Read the model definition and answer for the solid it produces. Units are mm, in the model's axes. A direction names the side the tool comes from. Give positions to 0.01 mm unless a question says otherwise; leave off trailing zeros. Order: outer loops, then holes, each group sorted by start corner. A loop starts at its lowest first (then second) coordinate and runs counter-clockwise, first axis right, second up. Notation, with made-up numbers: (72.5, 51.5) -> (116.5, 51.5) arc R21 cw to (116.5, 71.5) -> close; hole circle Ø10 at (-16, 63). An arc over 180 degrees is marked (long way). Use one line per item in the form item = value.
```python
from build123d import *

# Parameters (mm, degrees)
SKETCH1_W                                        = 183.850004878
SKETCH1_H                                        = 82.78473231
BOSS_EXTRUDE1_DEPTH                              = 30
CSK_FOR_M10_FLAT_HEAD_MACHINE_SCREW2_D           = 11
CSK_FOR_M10_FLAT_HEAD_MACHINE_SCREW2_CSINK_D     = 20
CSK_FOR_M10_FLAT_HEAD_MACHINE_SCREW2_CSINK_ANGLE = 80
CBORE_FOR_M8_HEX_HEAD_BOLT1_D                    = 9
CBORE_FOR_M8_HEX_HEAD_BOLT1_CBORE_D              = 18.01
CBORE_FOR_M8_HEX_HEAD_BOLT1_CBORE_DEPTH          = 5.68
MIRROR2_COPY_1_D                                 = 9
MIRROR2_COPY_1_CBORE_D                           = 18.01
MIRROR2_COPY_1_CBORE_DEPTH                       = 5.68
F_20_0MM_START                                   = 20
F_20_0MM_DOWEL_SLOT1_DEPTH                       = 10


# Read off the part's stored shape, not the designer's step: Ø20.0mm Dowel Slot1
with BuildPart() as part:
    # Sketch1 → Boss-Extrude1 (new body)
    with BuildSketch(Plane(origin=(0, 0, 0), x_dir=(1, 0, 0), z_dir=(0, 1, 0))):
        Rectangle(SKETCH1_W, SKETCH1_H)
    extrude(amount=BOSS_EXTRUDE1_DEPTH)

    # CSK for M10 Flat Head Machine Screw2 (through all)
    with Locations(Plane(origin=(0, 30, 0), x_dir=(1, 0, 0), z_dir=(0, 1, 0))):
        with Locations((0, 0)):
            CounterSinkHole(CSK_FOR_M10_FLAT_HEAD_MACHINE_SCREW2_D / 2, CSK_FOR_M10_FLAT_HEAD_MACHINE_SCREW2_CSINK_D / 2, counter_sink_angle=CSK_FOR_M10_FLAT_HEAD_MACHINE_SCREW2_CSINK_ANGLE)

    # CBORE for M8 Hex Head Bolt1 (through all)
    with Locations(Plane(origin=(-73.52781125, 30, -24.202787729), x_dir=(0, 0, 1), z_dir=(0, 1, 0))):
        with Locations((0, 0)):
            cbore_for_m8_hex_head_bolt1 = CounterBoreHole(CBORE_FOR_M8_HEX_HEAD_BOLT1_D / 2, CBORE_FOR_M8_HEX_HEAD_BOLT1_CBORE_D / 2, CBORE_FOR_M8_HEX_HEAD_BOLT1_CBORE_DEPTH)

    # Mirror1: CBORE for M8 Hex Head Bolt1 across plane
    add(cbore_for_m8_hex_head_bolt1.mirror(Plane.XY), mode=Mode.SUBTRACT)

    # Mirror2: CBORE for M8 Hex Head Bolt1 across plane
    add(cbore_for_m8_hex_head_bolt1.mirror(Plane(origin=(0, 0, 0), x_dir=(0, 0, 1), z_dir=(1, 0, 0))), mode=Mode.SUBTRACT)

    # Mirror2 copy 1 (through all)
    with Locations(Plane(origin=(73.52781125, 30, 24.202787729), x_dir=(0, 0, -1), z_dir=(0, 1, 0))):
        with Locations((0, 0)):
            CounterBoreHole(MIRROR2_COPY_1_D / 2, MIRROR2_COPY_1_CBORE_D / 2, MIRROR2_COPY_1_CBORE_DEPTH)

    # Ø20.0mm Dowel Slot1 outline → Ø20.0mm Dowel Slot1 (cut)
    with BuildSketch(Plane(origin=(0, 0, 0), x_dir=(1, 0, 0), z_dir=(0, 1, 0)).offset(F_20_0MM_START)):
        with BuildLine():
            Line((-50, -41.392366155), (50, -41.392366155))
            ThreePointArc((50, -41.392366155), (47.071067812, -34.321298343), (40, -31.392366155))
            Line((40, -31.392366155), (-40, -31.392366155))
            ThreePointArc((-40, -31.392366155), (-47.071067812, -34.321298343), (-50, -41.392366155))
        make_face()
    f_20_0mm_dowel_slot1 = extrude(amount=F_20_0MM_DOWEL_SLOT1_DEPTH, mode=Mode.SUBTRACT)

    # Mirror3: Ø20.0mm Dowel Slot1 across plane
    add(f_20_0mm_dowel_slot1.mirror(Plane.XY), mode=Mode.SUBTRACT)

    # Sketch20 → M12x1.5 Tapped Hole1 (revolve, cut)
    with BuildSketch(Plane(origin=(-33.179705033, 30, -12.1730736), x_dir=(0, 0, 1), z_dir=(1, 0, 0))):
        Polygon((0, 0), (0, 18.15451825), (5.25, 15), (5.25, 0), align=None)
    m12x1_5_tapped_hole1 = revolve(axis=Axis((-33.179705033, 36.35, -12.1730736), (0, -1, 0)), mode=Mode.SUBTRACT)

    # Mirror4: M12x1.5 Tapped Hole1 across plane
    add(m12x1_5_tapped_hole1.mirror(Plane.XY), mode=Mode.SUBTRACT)

    # Mirror5: M12x1.5 Tapped Hole1 across plane
    add(m12x1_5_tapped_hole1.mirror(Plane(origin=(0, 0, 0), x_dir=(0, 0, 1), z_dir=(1, 0, 0))), mode=Mode.SUBTRACT)

    # Mirror5 copy 1 sketch → Mirror5 copy 1 (revolve, cut)
    with BuildSketch(Plane(origin=(33.179705033, 30, 12.1730736), x_dir=(0, 0, -1), z_dir=(-1, 0, 0))):
        Polygon((0, 0), (0, 18.15451825), (5.25, 15), (5.25, 0), align=None)
    revolve(axis=Axis((33.179705033, 36.35, 12.1730736), (0, -1, 0)), mode=Mode.SUBTRACT)


solid = part.part
```
Item 1: Which of the six approach directions +Z, -Z, +X, -X, +Y, -Y give full straight-line access (tool end or side, diameter ignored) to faces 4 (the flat face through (-1, 20, -36)), 5 (the flat face through (-1, 0, -10)), 6 (the cylindrical face through (-46.99, 24.93, 34.24)), 7 (the cylindrical face through (31.169, 22.605, 7.323))?
Checks:
face_4 = -Z, +Y
face_5 = +Z, -Z, +X, -X, -Y
face_6 = +Z, +Y
face_7 = +Y
Item 2: Straight lines are drawn through the part: L1, parallel to X at y = 27.5, z = -23.5 (3 decimals); L2, parallel to Z at x = 0, y = 14; L3, parallel to Z at x = -29, y = 19.25. For each, find the intervals that lie inside material, in ascending order. Write a range as from..to.
Checks:
L1 = -91.925..-82.505, -64.55..64.55, 82.505..91.925
L2 = -41.39..-5.5, 5.5..41.39
L3 = -41.39..-15.35, -9..9, 15.35..41.39
Item 3: Given pin 1 Ø8 at (x, z) = (73.53, -24.2) entering from -Y; pin 2 Ø9 at (x, z) = (-72.5, -24) entering from +Y; pin 3 Ø3 at (x, z) = (11.5, 37) entering from +Y; pin 4 Ø5 at (x, y) = (10, 25.5) entering from +Z, each flat-ended and moving along its own axis, determine where each tip first touches the part or whether it passes through.
Checks:
pin_1 = through
pin_2 = 24.32
pin_3 = 20
pin_4 = 31.39
Item 4: The part is cut by section C-C on z = -27. Give the vertices of the cut face in (x, y) (3 decimals), and give its area (3 significant figures).
Checks:
outline = (-91.925, 0) -> (-77.053, 0) -> (-77.053, 24.32) -> (-82.087, 24.32) -> (-82.087, 30) -> (-91.925, 30) -> close; (-70.003, 0) -> (70.003, 0) -> (70.003, 24.32) -> (64.968, 24.32) -> (64.968, 30) -> (-64.968, 30) -> (-64.968, 24.32) -> (-70.003, 24.32) -> close; (77.053, 0) -> (91.925, 0) -> (91.925, 30) -> (82.087, 30) -> (82.087, 24.32) -> (77.053, 24.32) -> close
area = 4,980 mm²
Item 5: The part is cut by section A-A on z = 0. Give the vertices of the cut face in (x, y) (3 decimals), and give its area (3 significant figures).
Checks:
outline = (-91.925, 0) -> (-5.5, 0) -> (-5.5, 24.637) -> (-10, 30) -> (-91.925, 30) -> close; (5.5, 0) -> (91.925, 0) -> (91.925, 30) -> (10, 30) -> (5.5, 24.637) -> close
area = 5,160 mm²
Item 6: The part is cut by section D-D on y = 8. Give the vertices of the cut face in (x, z) (3 decimals), and give its area (3 significant figures).
Checks:
outline = (-91.925, -41.392) -> (91.925, -41.392) -> (91.925, 41.392) -> (-91.925, 41.392) -> close; hole circle Ø9 at (-73.528, -24.203); hole circle Ø9 at (-73.528, 24.203); hole circle Ø11 at (0, 0); hole circle Ø9 at (73.528, -24.203); hole circle Ø9 at (73.528, 24.203)
area = 14,900 mm²
Item 7: Determine the mould class of faces 1 (the flat face through (-22, 30, -1)), 2 (the cylindrical face through (-31.169, 22.605, 7.323)), 3 (the cylindrical face through (-46.99, 24.93, -34.24)) for opening direction Z: +Z half, -Z half, draft (parallel to the pull), parting line (faces both ways), or undercut.
Checks:
face_1 = draft
face_2 = undercut
face_3 = -Z half
Item 8: The part is cut by section B-B on x = 0. Give the vertices of the cut face in (y, z).
Checks:
outline = (0, -41.39) -> (20, -41.39) -> (20, -31.39) -> (30, -31.39) -> (30, -10) -> (24.64, -5.5) -> (0, -5.5) -> close; (0, 5.5) -> (24.64, 5.5) -> (30, 10) -> (30, 31.39) -> (20, 31.39) -> (20, 41.39) -> (0, 41.39) -> close
